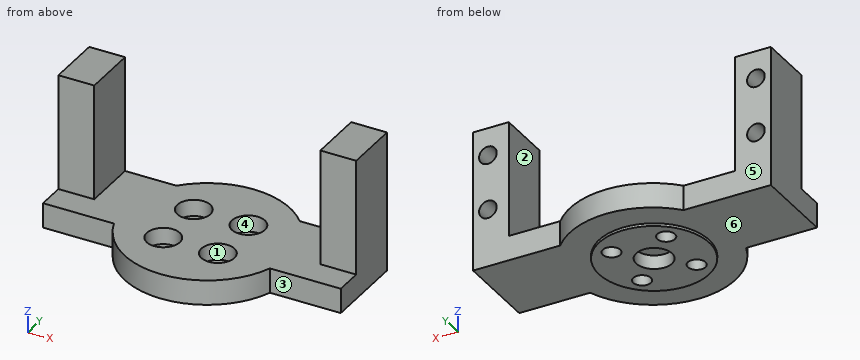
Autodesk Inventor part; units mm, degrees
ref_plane "工作平面1" through (0, 0, 0.5) normal (0, 0, -1) x (-1, 0, 0)
ref_plane "YZ Plane" through (0, 0, 0) normal (1, 0, 0) x (0, 1, 0)
ref_plane "XZ Plane" through (0, 0, 0) normal (0, 1, 0) x (-1, 0, 0)
sketch "草圖1" plane through (0, 0, 0) normal (0, 0, 1) x (1, 0, 0)
  circle A0 centre (0, 0) radius 10
  dimension "d0" = 20
extrude "擠出1" add sketch "草圖1" along normal blind 5
ref_plane "工作平面1" through (0, 0, 0.5) normal (0, 0, -1) x (-1, 0, 0)
sketch "草圖4" plane through (0, 0, 0.5) normal (0, 0, -1) x (-1, 0, 0)
  circle A0 centre (-0.2588, 0) radius 15
  point P0 (0, 0)
  dimension "d18" = 30
extrude "擠出3" add sketch "草圖4" against normal up to surface (4.5 mm away)
sketch "草圖2" plane through (0, 0, 5) normal (0, 0, 1) x (1, 0, 0)
  circle A0 centre (0, 0) radius 7
  line L0 (-4.9497, -4.9497) -> (4.9497, -4.9497)
  line L1 (4.9497, -4.9497) -> (4.9497, 4.9497)
  line L2 (4.9497, 4.9497) -> (-4.9497, 4.9497)
  line L3 (-4.9497, 4.9497) -> (-4.9497, -4.9497)
  line L4 (-4.9497, -4.9497) -> (4.9497, 4.9497) construction
  line L5 (4.9497, -4.9497) -> (-4.9497, 4.9497) construction
  dimension "d3" = 14
hole "孔1" at (4.9497, 4.9497, 5) at (-4.9497, 4.9497, 5) at (-4.9497, -4.9497, 5) at (4.9497, -4.9497, 5) direction (0, 0, -1) diameter 3.2 depth 8 tip angle 118 counterbore diameter 6 counterbore depth 3
sketch "草圖5" plane through (0.2588, 0, 5) normal (0, 0, 1) x (1, 0, 0)
  line L0 (-27, 10) -> (-10, 10)
  line L1 (-10, 10) -> (-10, -5)
  line L2 (-10, -5) -> (-27, -5)
  line L3 (-27, -5) -> (-27, 10)
  line L4 (10, 10) -> (27, 10)
  line L5 (27, 10) -> (27, -5)
  line L6 (27, -5) -> (10, -5)
  line L7 (10, -5) -> (10, 10)
  circle A0 centre (0, 0) radius 15
  point P0 (-0.2588, 0)
  dimension "d21" = 10
  dimension "d22" = 10
  dimension "d23" = 10
  dimension "d24" = 15
  dimension "d27" = 17
  dimension "d28" = 17
extrude "擠出4" add sketch "草圖5" against normal up to surface (4.5 mm away) contours L0 A0 L2 L3 | L0 L1 L2 A0 | A0 L6 L7 L4 | L4 L5 L6 A0
sketch "草圖6" plane through (0, 0, 5) normal (0, 0, 1) x (1, 0, 0)
  line L0 (-26.7412, 10) -> (-10.9215, 10)
  line L1 (-26.7412, 10) -> (-20.2412, 10)
  line L2 (-20.2412, 10) -> (-20.2412, 0)
  line L3 (-20.2412, 0) -> (-26.7412, 0)
  line L4 (-26.7412, 0) -> (-26.7412, 10)
  line L5 (27.2588, 10) -> (27.2588, -5)
  line L6 (27.2588, 10) -> (20.7588, 10)
  line L7 (20.7588, 10) -> (20.7588, 0)
  line L8 (20.7588, 0) -> (27.2588, 0)
  line L9 (27.2588, 0) -> (27.2588, 10)
  point P0 (0, 0)
  dimension "d29" = 41
  dimension "d30" = 10
  dimension "d31" = 10
extrude "擠出5" add sketch "草圖6" along normal blind 21
sketch "草圖7" plane through (-26.7412, 10, 0.5) normal (0, 1, 0) x (1, 0, 0)
  line L0 (2.7, -10.5) -> (51.3, -10.5)
  line L1 (51.3, -10.5) -> (51.3, -20.5)
  line L2 (51.3, -20.5) -> (2.7, -20.5)
  line L3 (2.7, -20.5) -> (2.7, -10.5)
  line L4 (0, 0) -> (0, -25.5)
  line L5 (6.5, -25.5) -> (0, -25.5)
  point P0 (26.7412, 0.5)
  dimension "d34" = 48.6
  dimension "d35" = 2.7
  dimension "d36" = 5
  dimension "d37" = 10
hole "孔2" at (-24.0412, 10, 21) at (-24.0412, 10, 11) at (24.5588, 10, 21) at (24.5588, 10, 11) direction (0, -1, 0) diameter 3.2 depth 8 tip angle 118
sketch "草圖8" plane through (0, 0, 0) normal (0, 0, -1) x (-1, 0, 0)
  circle A0 centre (0, 0) radius 3.25
  dimension "d45" = 6.5
extrude "擠出6" cut sketch "草圖8" against normal blind 2.5
properties part number "腕-2" material "熱塑性塑膠樹脂"
Geometry check sheet. Reference: the model listing, model coordinates, mm. Face numbers are marked on the shaded views. A direction names the side the tool comes from. Give positions to 0.01 mm unless a question says otherwise; leave off trailing zeros. Order: outer loops, then holes, each group sorted by start corner. A loop starts at its lowest first (then second) coordinate and runs counter-clockwise, first axis right, second up. Notation, with made-up numbers: (16, 80) - (26, 80) arc R19 ccw to (26, 104) - close; hole circle Ø4 at (64, 50.5). An arc over 180 degrees is marked (long way). Answer in a Markdown table with one row per item. Add a question column.
Q1. Cross-section at C-C, the plane y = -6. Enter the section's corners in (x, z).
Q2. Cross-section at A-A, the plane z = 17. Enter the section's corners in (x, y), then the cut area to 3 significant figures.
Q3. Gauge pin test, flat ends, axial feed: pin 1 (2 mm diameter, centred on x = 22.5, z = 13, fed in from -Y); pin 2 (8 mm diameter, centred on x = 16, y = -8.5, fed in from +Z); pin 3 (4 mm diameter, centred on x = 24.56, z = 21, fed in from +Y). Record the tip position at first contact, or that the pin passes through.
Q4. Mould release check, pull along Y, two halves, no side actions. Record for the marked faces 4, 5 and 6: pulls with the +Y half, pulls with the -Y half, needs draft (parallel to the pull), parting line crosses it, or undercut.
Q5. Cross-section at B-B, the plane y = 6. Count the separate pieces of the cut face and the enclosed holes in it, then the cut area to 3 significant figures.
Q6. Cross-section at D-D, the plane x = 0. Enter the section's corners in (y, z).
Q7. Material ranges on probe 1 along X at (y, z) = (6.5, 8); probe 2 along Y at (x, z) = (4.5, 1.75); probe 3 along Y at (x, z) = (0, 1.1), recorded low to high. Write a range as from..to.
Q8. Tool access check on the marked faces 1, 2 and 3. Record the directions out of +Z, -Z, +X, -X, +Y, -Y that give a thin tool (end or side, any length) a straight path to the whole face; none if there is none.
Check values:
| question | item | result |
|---|---|---|
| 1 | outline | (-13.49, 0.5) - (-8, 0.5) - (-8, 0) - (-6.16, 0) - (-6.16, 2) - (-7.76, 2) - (-7.76, 5) - (-13.49, 5) - close; (-3.74, 0) - (3.74, 0) - (3.74, 2) - (2.14, 2) - (2.14, 5) - (-2.14, 5) - (-2.14, 2) - (-3.74, 2) - close; (6.16, 0) - (8, 0) - (8, 0.5) - (14.01, 0.5) - (14.01, 5) - (7.76, 5) - (7.76, 2) - (6.16, 2) - close |
| 2 | outline | (-26.74, 0) - (-20.24, 0) - (-20.24, 10) - (-26.74, 10) - close; (20.76, 0) - (27.26, 0) - (27.26, 10) - (20.76, 10) - close |
| 2 | area | 130 mm^2 |
| 3 | pin 1 | stops at y = 0 |
| 3 | pin 2 | stops at z = 5 |
| 3 | pin 3 | stops at y = 10 |
| 4 | face 4 | undercut |
| 4 | face 5 | pulls with the +Y half |
| 4 | face 6 | needs draft |
| 5 | separate pieces | 3 |
| 5 | enclosed holes | 4 |
| 5 | area | 448 mm^2 |
| 6 | outline | (-15, 0.5) - (-10, 0.5) - (-10, 0) - (-3.25, 0) - (-3.25, 2.5) - (3.25, 2.5) - (3.25, 0) - (10, 0) - (10, 0.5) - (15, 0.5) - (15, 5) - (-15, 5) - close |
| 7 | probe 1 | x = -26.74..-20.24, 20.76..27.26 |
| 7 | probe 2 | y = -14.39..-6.49, -3.41..3.41, 6.49..14.39 |
| 7 | probe 3 | y = -15..-3.25, 3.25..15 |
| 8 | face 1 | +Z |
| 8 | face 2 | +Z, +Y, -Y |
| 8 | face 3 | +Z, -Z, +X, -Y |
